Model file for the job. Use its own axes, mm. Coordinates: 2 decimals unless noted, no trailing zeros. Order: outer loops, then holes, each group sorted by start corner. A loop starts at its lowest first (then second) coordinate and runs counter-clockwise, first axis right, second up. Notation, with made-up numbers: (36.5, 66) -> (76.5, 66) arc R23 ccw to (76.5, 82) -> close; hole circle Ø6 at (66.5, 9). An arc over 180 degrees is marked (long way). Return JSON: item names as keys, results as strings. Group by question number.
1) Probe line 1 (Y direction, x = 0, z = 2.15); line 2 (X direction, y = 57, z = 0.9). List the from-to ranges inside material, lowest first.
2) Cut at A-A (x = 0). Write the cut outline in (y, z).
3) Cut at C-C (y = 47). Write the cut outline in (x, z), and give its area (3 significant figures).
4) Pull direction X, two halves, no side cores. Call faces 1 (the cylindrical face through (-0.753, -72.224, 1.521)), 2 (the flat face through (0, 0, 0)): +X half, -X half, draft (parallel to the pull), parting line (faces both ways), or undercut.
5) Cut at B-B (z = 1.25). Write the cut outline in (x, y), and give its area (3 significant figures).
6) Flat gauge pins, fed straight in: pin 1 (1.5 mm diameter, centred on y = 35.5, z = 1, fed in from -X); pin 2 (0.9 mm diameter, centred on y = -27, z = 2, fed in from +X); pin 3 (0.9 mm diameter, centred on x = -51.5, z = 1.5, fed in from +Y). Where does each tip first touch, or does it go through?
from build123d import *

# Parameters (mm, degrees)
F0_W     = 150
F0_H     = 15
F1_DEPTH = 3
F2_W     = 15
F2_H     = 150
F3_DEPTH = 3
F4_R     = 3.475604
F5_DEPTH = 25


with BuildPart() as f1:
    # F0 (on Top) → F1 (new body)
    with BuildSketch(Plane.XY):
        Rectangle(F0_W, F0_H)
    extrude(amount=F1_DEPTH)

    # F2 (on Top) → F3 (join)
    with BuildSketch(Plane.XY):
        Rectangle(F2_W, F2_H)
    extrude(amount=F3_DEPTH)

    # F4 (on face) → F5 (cut)
    with BuildSketch(Plane.XY.offset(3)):
        with Locations((0, -68.830863)):
            Circle(F4_R)
    extrude(amount=-F5_DEPTH, mode=Mode.SUBTRACT)


solid = f1.part
Answers below:
{
 "1": {"line 1": "y = -75 to -72.31, -65.36 to 75", "line 2": "x = -7.5 to 7.5"},
 "2": {"outline": "(-75, 0) -> (-72.31, 0) -> (-72.31, 3) -> (-75, 3) -> close; (-65.36, 0) -> (75, 0) -> (75, 3) -> (-65.36, 3) -> close"},
 "3": {"outline": "(-7.5, 0) -> (7.5, 0) -> (7.5, 3) -> (-7.5, 3) -> close", "area": "45.0 mm^2"},
 "4": {"face 1": "undercut", "face 2": "draft"},
 "5": {"outline": "(-75, -7.5) -> (-7.5, -7.5) -> (-7.5, -75) -> (7.5, -75) -> (7.5, -7.5) -> (75, -7.5) -> (75, 7.5) -> (7.5, 7.5) -> (7.5, 75) -> (-7.5, 75) -> (-7.5, 7.5) -> (-75, 7.5) -> close; hole circle Ø6.95 at (0, -68.83)", "area": "4,240 mm^2"},
 "6": {"pin 1": "stops at x = -7.5", "pin 2": "stops at x = 7.5", "pin 3": "stops at y = 7.5"}
}
